from build123d import *

# Parameters (mm, degrees)
F0_W     = 50.8
F0_H     = 25.4
F0_W_2   = 47.625
F0_H_2   = 22.225
F1_DEPTH = 228.6
F2_R     = 2.5527
F3_DEPTH = 279.4
F4_R     = 2.5527
F5_DEPTH = 25.4


# Not quite as in the source:
# - a feature names something its author has since deleted; it is built from what else it names


with BuildPart() as f1:
    # F0 (on Front) → F1 (new body)
    with BuildSketch(Plane.XZ):
        Rectangle(F0_W, F0_H)
        Rectangle(F0_W_2, F0_H_2, mode=Mode.SUBTRACT)
    extrude(amount=F1_DEPTH)

    # F2 (on face) → F3 (cut)
    with BuildSketch(Plane(origin=(-25.4, 0, 0), x_dir=(0, -1, 0), z_dir=(-1, 0, 0))):
        with Locations((12.7, 0)):
            Circle(F2_R)
        with Locations((25.4, 0)):
            Circle(F2_R)
        with Locations((38.1, 0)):
            Circle(F2_R)
        with Locations((50.8, 0)):
            Circle(F2_R)
        with Locations((63.5, 0)):
            Circle(F2_R)
        with Locations((88.9, 0)):
            Circle(F2_R)
        with Locations((101.6, 0)):
            Circle(F2_R)
        with Locations((76.2, 0)):
            Circle(F2_R)
        with Locations((114.3, 0)):
            Circle(F2_R)
        with Locations((127, 0)):
            Circle(F2_R)
        with Locations((139.7, 0)):
            Circle(F2_R)
        with Locations((152.4, 0)):
            Circle(F2_R)
        with Locations((165.1, 0)):
            Circle(F2_R)
        with Locations((177.8, 0)):
            Circle(F2_R)
        with Locations((190.5, 0)):
            Circle(F2_R)
        with Locations((203.2, 0)):
            Circle(F2_R)
        with Locations((215.9, 0)):
            Circle(F2_R)
    extrude(amount=-F3_DEPTH, mode=Mode.SUBTRACT)

    # F4 (on face) → F5 (cut)
    with BuildSketch(Plane(origin=(0, 0, -12.7), x_dir=(1, 0, 0), z_dir=(0, 0, -1))):
        with Locations((12.7, 25.4)):
            Circle(F4_R)
        with Locations((-12.7, 25.4)):
            Circle(F4_R)
        with Locations((-12.7, 127)):
            Circle(F4_R)
        with Locations((-12.7, 101.6)):
            Circle(F4_R)
        with Locations((12.7, 152.4)):
            Circle(F4_R)
        with Locations((-12.7, 177.8)):
            Circle(F4_R)
        with Locations((12.7, 63.5)):
            Circle(F4_R)
        with Locations((12.7, 190.5)):
            Circle(F4_R)
        with Locations((12.7, 101.6)):
            Circle(F4_R)
        with Locations((-12.7, 76.2)):
            Circle(F4_R)
        with Locations((-12.7, 139.7)):
            Circle(F4_R)
        with Locations((12.7, 12.7)):
            Circle(F4_R)
        with Locations((12.7, 76.2)):
            Circle(F4_R)
        with Locations((12.7, 50.8)):
            Circle(F4_R)
        with Locations((12.7, 88.9)):
            Circle(F4_R)
        with Locations((12.7, 139.7)):
            Circle(F4_R)
        with Locations((12.7, 177.8)):
            Circle(F4_R)
        with Locations((12.7, 165.1)):
            Circle(F4_R)
        with Locations((-12.7, 190.5)):
            Circle(F4_R)
        with Locations((12.7, 38.1)):
            Circle(F4_R)
        with Locations((-12.7, 38.1)):
            Circle(F4_R)
        with Locations((12.7, 203.2)):
            Circle(F4_R)
        with Locations((-12.7, 63.5)):
            Circle(F4_R)
        with Locations((12.7, 127)):
            Circle(F4_R)
        with Locations((-12.7, 165.1)):
            Circle(F4_R)
        with Locations((-12.7, 88.9)):
            Circle(F4_R)
        with Locations((12.7, 114.3)):
            Circle(F4_R)
        with Locations((-12.7, 114.3)):
            Circle(F4_R)
        with Locations((-12.7, 152.4)):
            Circle(F4_R)
        with Locations((-12.7, 203.2)):
            Circle(F4_R)
        with Locations((-12.7, 12.7)):
            Circle(F4_R)
        with Locations((-12.7, 50.8)):
            Circle(F4_R)
        with Locations((12.7, 215.9)):
            Circle(F4_R)
        with Locations((-12.7, 215.9)):
            Circle(F4_R)
    extrude(amount=-F5_DEPTH, mode=Mode.SUBTRACT)


solid = f1.part
Here's how the part is built. I have some questions about the finished solid (model axes, mm). Round coordinates to 2 decimals unless told otherwise and drop trailing zeros. Loops run counter-clockwise (first coordinate to the right, second up) from the corner with the lowest first, then second, coordinate; pieces in that order, holes last. Notation, with made-up numbers: (47, -32.5) - (53, -32.5) arc R26 ccw to (53, -5.5) - close; hole circle Ø8 at (-25, 49). An arc over 180 degrees is marked (long way). One line per question, with ' | ' between items. Start each with the question number.
Q1. We'd pull the mould along Z, two halves only. Please class faces 1 (the cylindrical face through (-24.62, -187.95, 0.11)), 2 (the cylindrical face through (12.147, -188.008, -11.917)), 3 (the cylindrical face through (24.595, -205.635, 0.767)), 4 (the flat face through (0, -113, -12.7)): +Z half, -Z half, draft (parallel to the pull), parting line (faces both ways), or undercut.
Q2. I want a section at C-C (x = 21.5). Write out the boundary of the cut face in (y, z).
Q3. I want a section at A-A (z = -7.5). Write out the boundary of the cut face in (x, y), then the cut area to 3 significant figures.
Q4. Will this pin go through, and if not, where does the flat tip stop? pin 1 (3 mm diameter, centred on y = -76.2, z = 0, fed in from +X).
Q5. Please list where these lines run through material, in increasing order: line 1 (X direction, y = -114.3, z = -11.55); line 2 (X direction, y = -25.5, z = 4.25); line 3 (Z direction, x = 13, y = -99). Write a range as [from, to].
Q6. I want a section at D-D (y = -133.5). Write out the boundary of the cut face in (x, z).
Q7. I want a section at B-B (y = -165.1). State how many separate pieces and enclosed holes the cut face has, then the cut area to 3 significant figures.
Response values:
1) face 1: undercut | face 2: draft | face 3: undercut | face 4: -Z half
2) outline: (-228.6, -12.7) - (0, -12.7) - (0, -11.11) - (-228.6, -11.11) - close; (-228.6, 11.11) - (0, 11.11) - (0, 12.7) - (-228.6, 12.7) - close
3) outline: (-25.4, -228.6) - (-23.81, -228.6) - (-23.81, 0) - (-25.4, 0) - close; (23.81, -228.6) - (25.4, -228.6) - (25.4, 0) - (23.81, 0) - close | area: 726 mm²
4) pin 1: passes through
5) line 1: x = [-25.4, -15.25], [-10.15, 10.15], [15.25, 25.4] | line 2: x = [-25.4, -23.81], [23.81, 25.4] | line 3: z = [-12.7, -11.11], [11.11, 12.7]
6) outline: (-25.4, -12.7) - (25.4, -12.7) - (25.4, 12.7) - (-25.4, 12.7) - close; hole (-23.81, -11.11) - (23.81, -11.11) - (23.81, 11.11) - (-23.81, 11.11) - close
7) separate pieces: 6 | enclosed holes: 0 | area: 183 mm²
